Geometry check sheet. Reference: the model listing, model coordinates, mm. A direction names the side the tool comes from. Coordinates: 2 decimals unless noted, no trailing zeros. Loops run counter-clockwise (first coordinate to the right, second up) from the corner with the lowest first, then second, coordinate; pieces in that order, holes last.
from build123d import *

# Parameters (mm, degrees)
F1_DEPTH = 63.5
F2_DEPTH = 25.4
F3_DEPTH = 7.9375


with BuildPart() as f1:
    # F0 (on Front) → F1 (new body, symmetric)
    with BuildSketch(Plane.XZ):
        Polygon((-41.275, -9.525), (41.275, -9.525), (41.275, 9.525), (22.225, 9.525), (-41.275, 9.525), align=None)
    extrude(amount=F1_DEPTH, both=True)

    # F0 (on Front) → F2 (join, symmetric)
    with BuildSketch(Plane.XZ):
        with BuildLine():
            Line((22.225, 9.525), (41.275, 9.525))
            Line((41.275, 9.525), (41.275, 27.0002))
            ThreePointArc((41.275, 27.0002), (45.92468, 38.22552), (57.15, 42.8752))
            Line((57.15, 42.8752), (60.325, 42.8752))
            Line((60.325, 42.8752), (60.325, 61.9252))
            Line((60.325, 61.9252), (57.15, 61.9252))
            ThreePointArc((57.15, 61.9252), (32.454296, 51.695904), (22.225, 27.0002))
            Line((22.225, 27.0002), (22.225, 9.525))
        make_face()
    extrude(amount=F2_DEPTH, both=True)

    # F0 (on Front) → F3 (join, symmetric)
    with BuildSketch(Plane.XZ):
        with BuildLine():
            add(Edge.make_bspline(
                [(-41.275, 9.525), (-42.692475, 46.227396), (-4.809058, 62.667362), (57.15, 61.9252)],
                knots=[0, 0, 0, 0, 111.504536, 111.504536, 111.504536, 111.504536], degree=3))
            Line((-41.275, 9.525), (22.225, 9.525))
            Line((22.225, 9.525), (22.225, 27.0002))
            ThreePointArc((22.225, 27.0002), (32.454296, 51.695904), (57.15, 61.9252))
        make_face()
    extrude(amount=F3_DEPTH, both=True)


solid = f1.part
(1) Sectioned sample at B-B on y = -35.5. Record the cut outline in (x, z) (3 decimals), and give its area (3 significant figures).
Findings:
outline: (-41.275, -9.525) - (41.275, -9.525) - (41.275, 9.525) - (-41.275, 9.525) - close
area: 1,570 mm2
(2) Scan lines: L1, parallel to X at y = 22.5, z = 20.5 (3 decimals); L2, parallel to Y at x = -13.5, z = 29; L3, parallel to Z at x = -19, y = 54.5 (3 decimals). Record each from-to range of solid material in increasing order.
Findings:
L1: x = 22.225 to 41.275
L2: y = -7.94 to 7.94
L3: z = -9.525 to 9.525
(3) Gauge pin test, flat ends, axial feed: pin 1 Ø6 at (y, z) = (44.5, 5) entering from +X (3 decimals); pin 2 Ø19 at (x, z) = (48.5, 41.5) entering from +Y; pin 3 Ø5 at (y, z) = (-19.5, 21.5) entering from -X (3 decimals). Record the tip position at first contact, or that the pin passes through.
Findings:
pin 1: stops at x = 41.275
pin 2: stops at y = 25.4
pin 3: stops at x = 22.225
(4) Access from +Z, -Z, +X, -X, +Y, -Y to the whole of each face (thin tool, end or side, straight path). Record for faces 1 (the cylindrical face through (32.73, 16.55, 51.97)), 2 (the flat face through (59, 0, 42.875)), 3 (the flat face through (37, 25.4, 36)), 4 (the cylindrical face through (32.73, -16.79, 51.97)).
Findings:
face 1: +Z, -X, +Y
face 2: -Z, +X, +Y, -Y
face 3: +Z, +X, -X, +Y
face 4: +Z, -X, -Y
(5) Sectioned sample at A-A on y = 11.5. Record the cut outline in (x, z) (3 decimals).
Findings:
outline: (-41.275, -9.525) - (41.275, -9.525) - (41.275, 27) arc R15.875 cw to (57.15, 42.875) - (60.325, 42.875) - (60.325, 61.925) - (57.15, 61.925) arc R34.925 ccw to (22.225, 27) - (22.225, 9.525) - (-41.275, 9.525) - close
